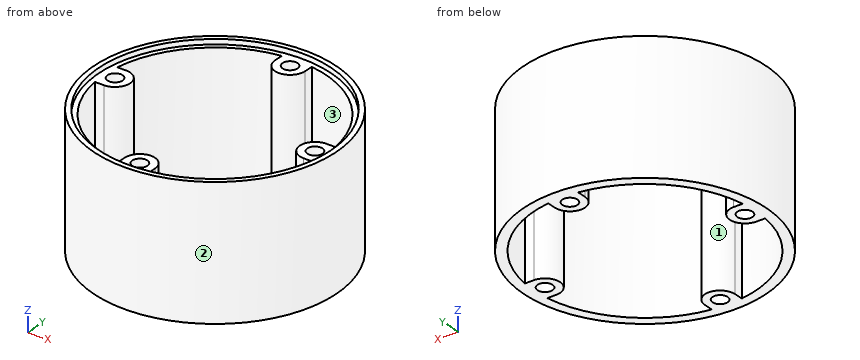
from build123d import *

# Parameters (mm, degrees)
SKETCH002_R        = 1.5
PAD_DEPTH          = 25
POLARPATTERN_COUNT = 4


with BuildPart() as part:
    # Sketch → Revolution (revolve)
    with BuildSketch(Plane.XZ):
        Polygon((24, 0), (24, 26), (23, 26), (23, 25), (22, 25), (22, 0), align=None)
    revolve(axis=Axis((0, 0, 0), (0, 0, 1)))

    # Sketch002 → Pad (new body)
    with BuildSketch(Plane(origin=(0, 0, 25), x_dir=(-1, 0, 0), z_dir=(0, 0, 1))):
        with BuildLine():
            Line((-3, 22), (-3, 20))
            ThreePointArc((-3, 20), (0, 17), (3, 20))
            Line((3, 20), (3, 22))
            Line((-3, 22), (3, 22))
        make_face()
        with Locations((0, 20)):
            Circle(SKETCH002_R, mode=Mode.SUBTRACT)
    pad = extrude(amount=-PAD_DEPTH)

    # PolarPattern: Pad ×4 about axis
    polarpattern_axis = Axis((0, 0, 25), (0, 0, 1))
    for i in range(1, POLARPATTERN_COUNT):
        add(pad.rotate(polarpattern_axis, i * 360 / POLARPATTERN_COUNT))


solid = part.part
Check sheet for the modelled part. Datum: model origin and axes. Units: mm. Face numbers are marked on the shaded views. Round coordinates to 2 decimals unless told otherwise and drop trailing zeros. Loops run counter-clockwise (first coordinate to the right, second up) from the corner with the lowest first, then second, coordinate; pieces in that order, holes last.
1. Gauge pin test, flat ends, axial feed: pin 1 Ø8 at (y, z) = (-16.5, 21) entering from -X; pin 2 Ø1.8 at (x, y) = (20, 0) entering from -Z (3 decimals); pin 3 Ø0.9 at (y, z) = (21, 6.5) entering from +X; pin 4 Ø5 at (y, z) = (-16, 4) entering from +X. Record the tip position at first contact, or that the pin passes through.
2. Sectioned sample at A-A on x = 0. Record the boundary of the cut face in (y, z).
3. Scan lines: probe 1 along Y at (x, z) = (0, 17); probe 2 along X at (y, z) = (19, 10); probe 3 along Z at (x, y) = (1.5, 19.5). Record each from-to range of solid material in increasing order.
4. Mould release check, pull along X, two halves, no side actions. Record for the marked faces 1, 2 and 3: released by +X, released by -X, zero draft, split by the parting line, or undercut.
5. Sectioned sample at D-D on x = -10.5. Record the boundary of the cut face in (y, z), and give its area (3 significant figures).
6. Sectioned sample at C-C on z = 19. Record the boundary of the cut face in (x, y), and give its area (3 significant figures).
Recorded:
1. pin 1: stops at x = -20.49
1. pin 2: passes through
1. pin 3: stops at x = 12.4
1. pin 4: stops at x = 19.84
2. outline: (-24, 0) - (-21.5, 0) - (-21.5, 25) - (-23, 25) - (-23, 26) - (-24, 26) - close; (-18.5, 0) - (-17, 0) - (-17, 25) - (-18.5, 25) - close; (17, 0) - (18.5, 0) - (18.5, 25) - (17, 25) - close; (21.5, 0) - (24, 0) - (24, 26) - (23, 26) - (23, 25) - (21.5, 25) - close
3. probe 1: y = -24 to -21.5, -18.5 to -17, 17 to 18.5, 21.5 to 24
3. probe 2: x = -14.66 to -11.09, -2.83 to -1.12, 1.12 to 2.83, 11.09 to 14.66
3. probe 3: z = 0 to 25
4. face 1: undercut
4. face 2: split by the parting line
4. face 3: undercut
5. outline: (-21.58, 0) - (-19.33, 0) - (-19.33, 25) - (-20.46, 25) - (-20.46, 26) - (-21.58, 26) - close; (19.33, 0) - (21.58, 0) - (21.58, 26) - (20.46, 26) - (20.46, 25) - (19.33, 25) - close
5. area: 115 mm2
6. outline: circle Ø48 at (0, 0); hole (-21.79, -3) arc R22 ccw to (-3, -21.79) - (-3, -20) arc R3 cw to (3, -20) - (3, -21.79) arc R22 ccw to (21.79, -3) - (20, -3) arc R3 cw to (20, 3) - (21.79, 3) arc R22 ccw to (3, 21.79) - (3, 20) arc R3 cw to (-3, 20) - (-3, 21.79) arc R22 ccw to (-21.79, 3) - (-20, 3) arc R3 cw to (-20, -3) - close; hole circle Ø3 at (-20, 0); hole circle Ø3 at (0, -20); hole circle Ø3 at (0, 20); hole circle Ø3 at (20, 0)
6. area: 364 mm2
